The listing builds one solid part. Answer for the finished solid, in the listing's coordinates (mm). Face numbers are marked on the shaded views. A direction names the side the tool comes from. Coordinates: 2 decimals unless noted, no trailing zeros. Write each loop counter-clockwise with the first axis right and the second up, starting at its lowest first coordinate (ties: lowest second). Pieces come first, ordered by that corner, then holes.
from build123d import *

# Parameters (mm, degrees)
BOSS_EXTRUDE2_DEPTH = 431.8
SKETCH8_R           = 3.175
CUT_EXTRUDE6_DEPTH  = 2.54


with BuildPart() as part:
    # Sketch3 → Boss-Extrude2 (new body)
    with BuildSketch(Plane.XY):
        Polygon((0, 0), (0, 1.5875), (49.2125, 1.5875), (49.2125, 50.8), (50.8, 50.8), (50.8, 0), align=None)
    extrude(amount=BOSS_EXTRUDE2_DEPTH)

    # Sketch8 → Cut-Extrude6 (cut)
    with BuildSketch(Plane(origin=(50.8, 0, 0), x_dir=(0, 0, -1), z_dir=(1, 0, 0))):
        with Locations((-29.464, 26.416)):
            Circle(SKETCH8_R)
        with BuildLine():
            Line((-254.508, 12.7), (-383.032, 12.7))
            ThreePointArc((-383.032, 12.7), (-397.256, 26.924), (-383.032, 41.148))
            Line((-383.032, 41.148), (-254.508, 41.148))
            ThreePointArc((-254.508, 41.148), (-240.284, 26.924), (-254.508, 12.7))
        make_face()
    extrude(amount=-CUT_EXTRUDE6_DEPTH, mode=Mode.SUBTRACT)


solid = part.part
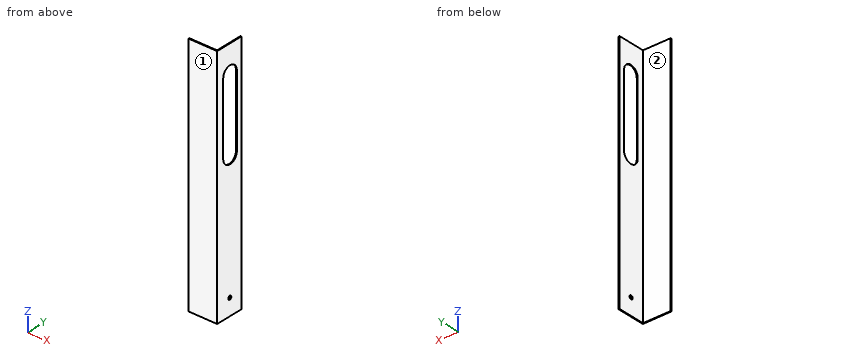
1. Flat-ended cylindrical pins translate along their axes: P1, Ø6, axis at y = 37, z = 47.5, coming from the -X side; P2, Ø1.5, axis at x = 6, z = 274.5, coming from the +Y side. Find the tip coordinate at first contact, or state that the pin passes through.
Results found:
P1: stops at x = 49.21
P2: stops at y = 1.59
2. Section C-C on z = 169 is taken. Give the vertices of the cut face in (x, y).
Results found:
outline: (0, 0) - (50.8, 0) - (50.8, 50.8) - (49.21, 50.8) - (49.21, 1.59) - (0, 1.59) - close
3. Find the intervals of material crossed by L1, parallel to Y at x = 42, z = 296.5; L2, parallel to X at y = 45.5, z = 155, in increasing order.
Results found:
L1: y = 0 to 1.59
L2: x = 49.21 to 50.8
4. Section A-A on z = 336 is taken. Give the vertices of the cut face in (x, y).
Results found:
outline: (0, 0) - (50.8, 0) - (50.8, 12.7) - (49.21, 12.7) - (49.21, 1.59) - (0, 1.59) - close; (49.21, 41.15) - (50.8, 41.15) - (50.8, 50.8) - (49.21, 50.8) - close
5. Section B-B on y = 36 is taken. Give the vertices of the cut face in (x, z), then the cut area to 3 significant figures.
Results found:
outline: (49.21, 0) - (50.8, 0) - (50.8, 243.56) - (49.21, 243.56) - close; (49.21, 393.98) - (50.8, 393.98) - (50.8, 431.8) - (49.21, 431.8) - close
area: 447 mm2
6. A tool of negligible diameter and unlimited length cuts with its end or side. For the marked faces 1 and 2, from which of +Z, -Z, +X, -X, +Y, -Y can it reach the whole face along a straight path? Write none if from no direction.
Results found:
face 1: +Z, -Z, +X, -X, -Y
face 2: +Z, -Z, -X, +Y
7. Section D-D on x = 30.5 is taken. Give the vertices of the cut face in (y, z), then the cut area to 3 significant figures.
Results found:
outline: (0, 0) - (1.59, 0) - (1.59, 431.8) - (0, 431.8) - close
area: 685 mm2
